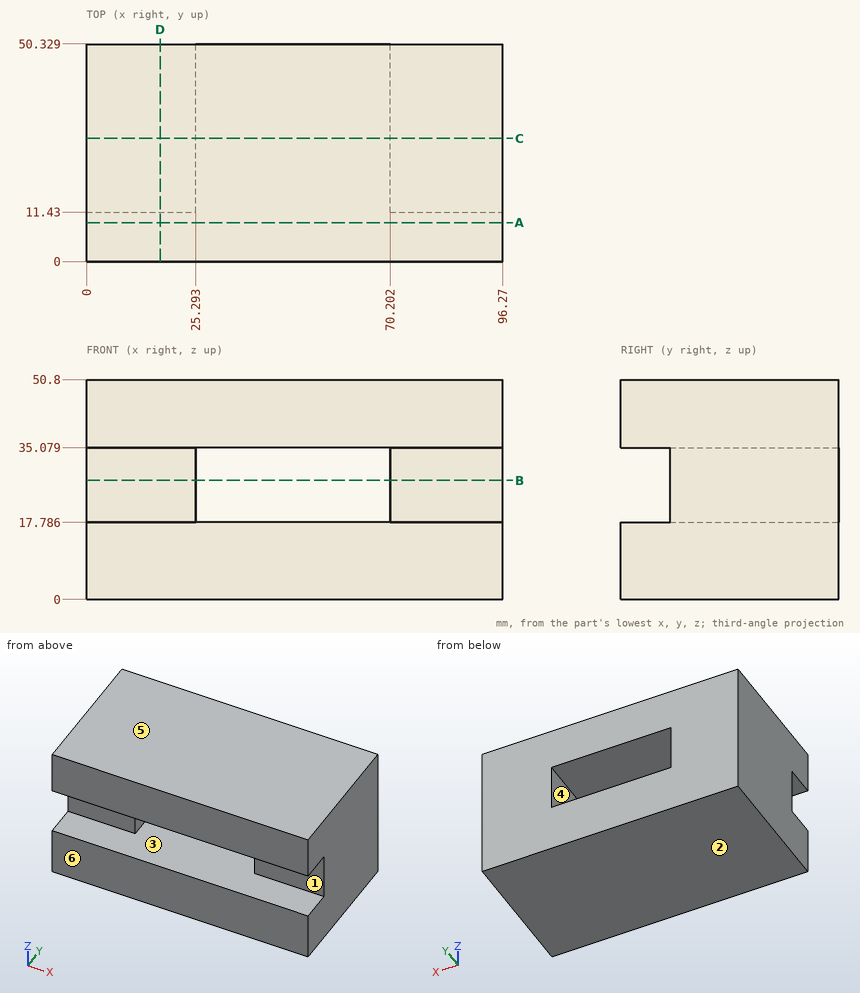
Geometry: see drawing. Coordinates: mm, zero at the bounding-box minimum. A direction names the side the tool comes from. Give positions to 0.01 mm unless a question says otherwise; leave off trailing zeros. Loops run counter-clockwise (first coordinate to the right, second up) from the corner with the lowest first, then second, coordinate; pieces in that order, holes last. Notation, with made-up numbers: (-3, 37) - (54, 37) arc R29 ccw to (54, 60) - close; hole circle Ø8 at (78, -24). An arc over 180 degrees is marked (long way). Use CSV: the item, a comma, the result in double quotes. Start each with the question number.
Item 1: Reachability of the marked faces 1, 2 and 3 from +Z, -Z, +X, -X, +Y, -Y: full face, straight path, thin tool, end or side. Return the list, or none.
Item 2: Section B-B on z = 27.5. Return loops of the section in (x, y).
Item 3: Line query: line 1 (X direction, y = 38, z = 34); line 2 (Z direction, x = 19.5, y = 11); line 3 (Y direction, x = 75.5, z = 18). Output: solid intervals per line, ascending.
Item 4: Section C-C on y = 28.5. Return loops of the section in (x, z).
Item 5: Mould query, pull axis Z, two halves, no side actions, for the marked faces 4, 5 and 6. Classes: pulls with the +Z half, pulls with the -Z half, needs draft (parallel to the pull), parting line crosses it, or undercut.
Item 6: Section D-D on x = 17. Return loops of the section in (y, z), then the cut area to 3 significant figures.
Item 7: Section A-A on y = 9. Return loops of the section in (x, z).
Item 8: Contact query for a flat-ended pin moving along its axis: P1, Ø8.5, axis at x = 7, z = 29, coming from the -Y side. Output: stop coordinate, or through.
Ans:
1,face 1,"+X, -X, -Y"
1,face 2,"-Z, +X, -X, +Y, -Y"
1,face 3,"-Y"
2,outline,"(0, 11.43) - (25.29, 11.43) - (25.29, 50.33) - (0, 50.33) - close; (70.2, 11.43) - (96.27, 11.43) - (96.27, 50.33) - (70.2, 50.33) - close"
3,line 1,"x = 0 to 25.29, 70.2 to 96.27"
3,line 2,"z = 0 to 17.79, 35.08 to 50.8"
3,line 3,"y = 11.43 to 50.33"
4,outline,"(0, 0) - (96.27, 0) - (96.27, 50.8) - (0, 50.8) - close; hole (25.29, 17.79) - (70.2, 17.79) - (70.2, 35.08) - (25.29, 35.08) - close"
5,face 4,"undercut"
5,face 5,"pulls with the +Z half"
5,face 6,"needs draft"
6,outline,"(0, 0) - (50.33, 0) - (50.33, 50.8) - (0, 50.8) - (0, 35.08) - (11.43, 35.08) - (11.43, 17.79) - (0, 17.79) - close"
6,area,"2,360 mm2"
7,outline,"(0, 0) - (96.27, 0) - (96.27, 17.79) - (0, 17.79) - close; (0, 35.08) - (96.27, 35.08) - (96.27, 50.8) - (0, 50.8) - close"
8,P1,"stops at y = 11.43"
